For this review, take the finished solid that the model builds, in its own axes (mm). A direction names the side the tool comes from. Round coordinates to 2 decimals unless told otherwise and drop trailing zeros. Order: outer loops, then holes, each group sorted by start corner. A loop starts at its lowest first (then second) coordinate and runs counter-clockwise, first axis right, second up. Notation, with made-up numbers: (66.5, 4) - (111.5, 4) arc R26 cw to (111.5, 21) - close; hole circle Ø2 at (78, 15.5). An arc over 180 degrees is marked (long way). Write each question's results on one line, items separated by ' | '. Start each with the question number.
(1) Take a section at C-C, the plane x = 0. Give the boundary of the cut face in (y, z).
(2) For faces 5 (the cylindrical face through (-7.493, -0.33, 14.93)), 6 (the flat face through (0, 0, 15)), 7 (the flat face through (137.5, -41, 69)), list the 3-axis set-ups (+Z, -Z, +X, -X, +Y, -Y) from which the entire face can be reached by the end or side of a thin tool; tool diameter is ignored.
(3) Insertion check: pin 1 Ø16.5 at (x, y) = (1.5, 1) entering from +Z; pin 2 Ø5 at (x, y) = (0, 0) entering from -Z; pin 3 Ø3 at (x, y) = (80, -33) entering from +Z; pin 4 Ø10.5 at (y, z) = (-50, 80) entering from +X. Each pin has a flat end and moves straight along its axis. Give the tip position at first contact, or say it passes through.
(4) Take a section at B-B, the plane y = -85.5. Give the boundary of the cut face in (x, z).
(5) For L1, parallel to X at y = -26.5, z = 84; L2, parallel to Z at x = 31.5, y = -24; L3, parallel to Y at x = 141, z = 80, list the stretches that pass through material, from the lowest coordinate up. Write a range as from..to.
(6) Take a section at D-D, the plane z = 80. Give the boundary of the cut face in (x, y).
(7) Draft analysis for pull direction Y (two halves, no side actions). For faces 1 (the flat face through (-2, 9, 10)), 2 (the cylindrical face through (-142.43, -77.553, 121.723)), 3 (the flat face through (142.57, 21.87, 57.14)), 4 (the cylindrical face through (-3, 0, 7)), state which applies: pulls with the +Y half, pulls with the -Y half, needs draft (parallel to the pull), parting line crosses it, or undercut.
(8) Take a section at A-A, the plane z = 118.5. Give the boundary of the cut face in (x, y).
Autodesk Inventor part; units mm, degrees
ref_plane "Work Plane1" through (0, 0, 10) normal (0, 0, 1) x (1, 0, 0)
ref_plane "YZ Plane" through (0, 0, 0) normal (1, 0, 0) x (0, 1, 0)
ref_plane "XZ Plane" through (0, 0, 0) normal (0, 1, 0) x (-1, 0, 0)
sketch "Sketch1" plane through (0, 0, 0) normal (0, 0, 1) x (1, 0, 0)
  line L0 (-147.5, -50) -> (147.5, -50)
  line L1 (147.5, -50) -> (147.5, 50)
  line L2 (147.5, 50) -> (-147.5, 50)
  line L3 (-147.5, 50) -> (-147.5, -50)
  line L4 (-147.5, -50) -> (147.5, 50) construction
  line L5 (147.5, -50) -> (-147.5, 50) construction
  point P0 (0, 0)
  dimension "d0" = 295
  dimension "d1" = 100
extrude "Extrusion1" add sketch "Sketch1" along normal blind 10
sketch "Sketch2" plane through (0, 0, 10) normal (0, 0, 1) x (1, 0, 0)
  circle A0 centre (0, 0) radius 3
  dimension "d13" = 6
extrude "Extrusion2" cut sketch "Sketch2" against normal through all
sketch "Sketch4" plane through (147.5, -50, 0) normal (1, 0, 0) x (0, 0, -1)
  circle A0 centre (-80, 0) radius 50 construction
  line L0 (0, 0) -> (-10, 0)
  line L1 (0, 0) -> (-48.75, -39.0312)
  line L2 (-10, 0) -> (-10, 100)
  line L3 (-10, 100) -> (-105.6226, 42.9358)
  arc A1 (-105.6226, 42.9358) -> (-48.75, -39.0312) centre (-80, 0) ccw
  line L4 (0, 0) -> (-10, 0)
  line L5 (-10, 100) -> (-10, 0)
  dimension "d8" = 100
  dimension "d20" = 80
extrude "Extrusion3" add sketch "Sketch4" against normal blind 295
ref_plane "Work Plane1" through (0, 0, 10) normal (0, 0, 1) x (1, 0, 0)
sketch "Sketch5" plane through (0, 0, 10) normal (0, 0, 1) x (1, 0, 0)
  line L0 (147.5, 50) -> (-147.5, 50)
  line L1 (147.5, -100) -> (-147.5, -100)
  line L2 (-137.5, 50) -> (137.5, 50)
  line L3 (137.5, 50) -> (137.5, -100)
  line L4 (137.5, -100) -> (-137.5, -100)
  line L5 (-137.5, -100) -> (-137.5, 50)
  line L6 (-147.5, 50) -> (-147.5, -50)
  line L7 (147.5, -50) -> (147.5, 50)
  point P0 (0, 0)
  dimension "d16" = 10
  dimension "d17" = 10
extrude "Extrusion4" cut sketch "Sketch5" along normal through all
sketch "Sketch7" plane through (0, 0, 10) normal (0, 0, 1) x (1, 0, 0)
  circle A0 centre (0, 0) radius 3
  circle A1 centre (0, 0) radius 7.5
  dimension "d23" = 15
extrude "Extrusion6" add sketch "Sketch7" along normal blind 5
sketch "Sketch8" plane through (0, 0, 15) normal (0, 0, 1) x (1, 0, 0)
  circle A0 centre (0, 0) radius 7.5
extrude "Extrusion7" add sketch "Sketch8" along normal blind 5
sketch "Sketch9" plane through (147.5, -50, 0) normal (1, 0, 0) x (0, 0, -1)
  arc A0 (-105.6226, 42.9358) -> (-48.75, -39.0312) centre (-80, 0) ccw
  circle A1 centre (-80, 0) radius 4
  point P0 (0, 50)
  dimension "d28" = 8
extrude "Extrusion8" cut sketch "Sketch9" against normal through all
properties part number "HA004"
Results below:
1) outline: (-58.01, 10) - (-50, 0) - (-3, 0) - (-3, 15) - (3, 15) - (3, 0) - (50, 0) - (50, 10) - (7.5, 10) - (7.5, 20) - (-7.5, 20) - (-7.5, 10) - close
2) face 5: +Z | face 6: -Z | face 7: +Z, +Y, -Y
3) pin 1: stops at z = 20 | pin 2: stops at z = 15 | pin 3: stops at z = 10 | pin 4: stops at x = 147.5
4) outline: (-147.5, 44.34) - (-137.5, 44.34) - (-137.5, 115.21) - (-147.5, 115.21) - close; (137.5, 44.34) - (147.5, 44.34) - (147.5, 115.21) - (137.5, 115.21) - close
5) L1: x = -147.5..-137.5, 137.5..147.5 | L2: z = 0..10 | L3: y = -100..-54, -46..8.23
6) outline: (-147.5, -100) - (-137.5, -100) - (-137.5, -54) - (-147.5, -54) - close; (-147.5, -46) - (-137.5, -46) - (-137.5, 8.23) - (-147.5, 8.23) - close; (137.5, -100) - (147.5, -100) - (147.5, -54) - (137.5, -54) - close; (137.5, -46) - (147.5, -46) - (147.5, 8.23) - (137.5, 8.23) - close
7) face 1: needs draft | face 2: parting line crosses it | face 3: pulls with the +Y half | face 4: undercut
8) outline: (-147.5, -81.9) - (-137.5, -81.9) - (-137.5, -18.1) - (-147.5, -18.1) - close; (137.5, -81.9) - (147.5, -81.9) - (147.5, -18.1) - (137.5, -18.1) - close
